Geometry: see drawing. Coordinates: mm, zero at the bounding-box minimum. A direction names the side the tool comes from. Coordinates: 2 decimals unless noted, no trailing zeros. Order: outer loops, then holes, each group sorted by start corner. A loop starts at its lowest first (then second) coordinate and runs counter-clockwise, first axis right, second up. Notation, with made-up numbers: (80.25, 5.25) -> (134.25, 5.25) arc R7 ccw to (134.25, 15.25) -> close; hole circle Ø5 at (71.5, 80.5). An arc over 180 degrees is marked (long way). Use one line per item in the form item = value.
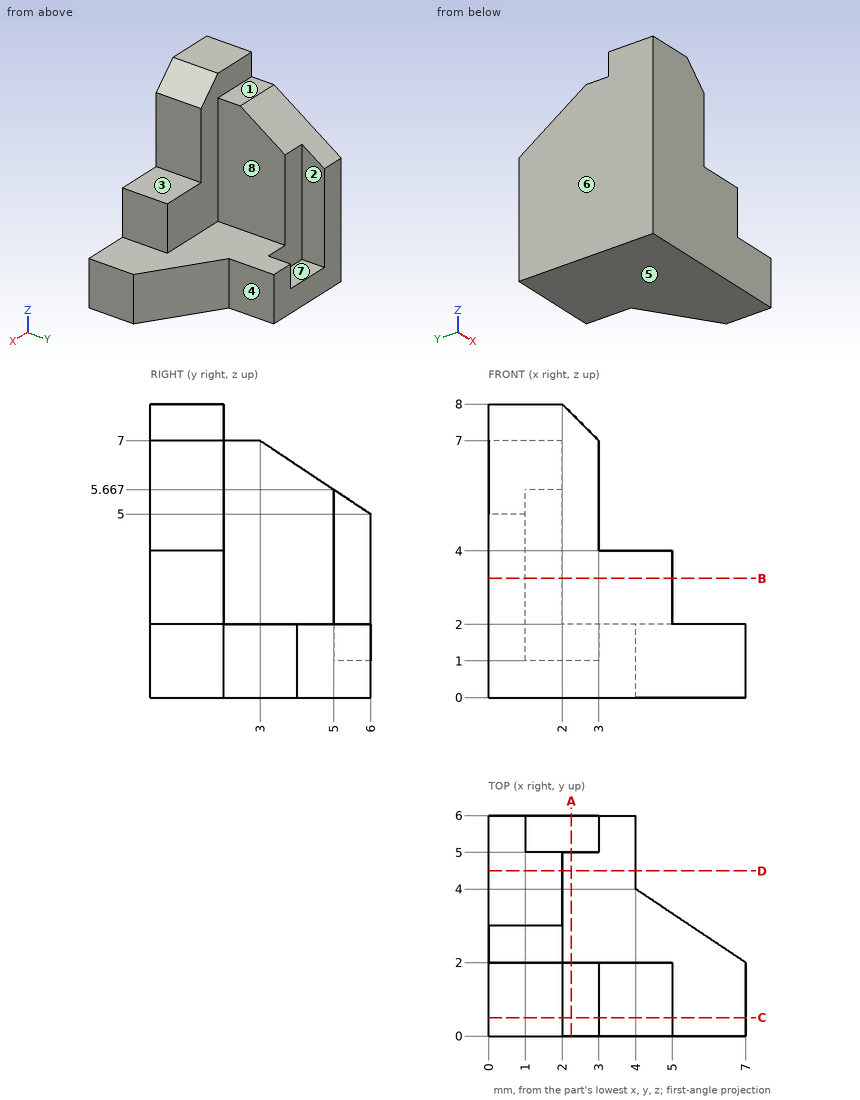
1) Section C-C, the plane y = 0.5. Output: boundary loops of the cut face in (x, z), and give its area (3 significant figures).
Results found:
outline = (0, 0) -> (7, 0) -> (7, 2) -> (5, 2) -> (5, 4) -> (3, 4) -> (3, 7) -> (2, 8) -> (0, 8) -> close
area = 35.5 mm2
2) Access query for the marked faces 1, 2, 3, 4 and 5. Directions: +Z, -Z, +X, -X, +Y, -Y. A direction counts if a zero-diameter tool reaches every point of the face in a straight line with its end or side. Return the directions, or none.
Results found:
face_1 = +Z, +X, -X, +Y
face_2 = +Z, +Y
face_3 = +Z, +X, +Y, -Y
face_4 = +Z, -Z, +X, +Y
face_5 = -Z, +X, -X, +Y, -Y
3) Section A-A, the plane x = 2.25. Output: boundary loops of the cut face in (y, z), and give its area (3 significant figures).
Results found:
outline = (0, 0) -> (6, 0) -> (6, 1) -> (5, 1) -> (5, 2) -> (2, 2) -> (2, 7.75) -> (0, 7.75) -> close
area = 22.5 mm2
4) Section B-B, the plane z = 3.25. Output: boundary loops of the cut face in (x, y).
Results found:
outline = (0, 0) -> (5, 0) -> (5, 2) -> (2, 2) -> (2, 5) -> (1, 5) -> (1, 6) -> (0, 6) -> close
5) Section D-D, the plane y = 4.5. Output: boundary loops of the cut face in (x, z).
Results found:
outline = (0, 0) -> (4, 0) -> (4, 2) -> (2, 2) -> (2, 6) -> (0, 6) -> close
6) Material intervals for probe 1 along Y at (x, z) = (5.5, 1); probe 2 along X at (y, z) = (5.75, 3); probe 3 along Z at (x, y) = (3.25, 1), sorted ascending. Write a range as from..to.
Results found:
probe_1 = 0..3
probe_2 = 0..1
probe_3 = 0..4
7) Contact query for flat-ended pins moving along their axis: P1, Ø1, axis at y = 0.5, z = 3, coming from the +X side; P2, Ø1, axis at x = 2, z = 5.5, coming from the +Y side; P3, Ø1, axis at x = 4.5, y = 1, coming from the +Z side. Output: stop coordinate, or through.
Results found:
P1 = 5
P2 = 5
P3 = 4
8) Pull-direction query (X, two-part tool) for the marked faces 6, 7 and 8; classes: released by +X, released by -X, zero draft, split by the parting line, or undercut.
Results found:
face_6 = released by -X
face_7 = undercut
face_8 = released by +X
